Part model, mm, in its own coordinate system. A direction names the side the tool comes from. Give positions to 0.01 mm unless a question says otherwise; leave off trailing zeros. Write each loop counter-clockwise with the first axis right and the second up, starting at its lowest first coordinate (ties: lowest second). Pieces come first, ordered by that corner, then holes. Notation, with made-up numbers: M 13,40.25 L 57,40.25 A18 cw 57,74.25 Z; hole C 2,47 d1. An arc over 180 degrees is marked long. Answer as CSV lines item,"result". Start each with the question number.
Item 1: Band-saw the part on A-A, the plane x = -13.5. List the corners of the cut face in (y, z), then the cut area to 3 significant figures.
Item 2: Pin check, flat tips, straight feed: pin 1 (1 mm diameter, centred on x = -52.5, z = -3.5, fed in from +Y); pin 2 (0.5 mm diameter, centred on x = -25.5, z = -3.5, fed in from -Y); pin 3 (11.5 mm diameter, centred on x = -26, y = -10.5, fed in from +Z); pin 4 (0.6 mm diameter, centred on x = -25, y = 8.5, fed in from +Z). Stop position of each tip, or through.
Item 3: Two-plate mould, pull along Z, no slides. Class faces 1 (the flat face through (-52.292, -33.704, -1.014)), 2 (the flat face through (-27, 17, -2)), 3 (the flat face through (-68, 13, -4)): +Z half, -Z half, draft (parallel to the pull), parting line (faces both ways), or undercut.
Item 4: Band-saw the part on C-C, the plane y = 13. List the corners of the cut face in (x, z).
Item 5: Wall check: L1, parallel to X at y = -2, z = -2.35; L2, parallel to Y at x = -34, z = -2; L3, parallel to Y at x = -32.5, z = -1.25. Give the ranges that are in metal, low to high. Write a range as from..to.
Item 6: Band-saw the part on D-D, the plane y = -18.5. List the corners of the cut face in (x, z), then the cut area to 3 significant figures.
Item 7: 3-axis set-ups, long thin cutter, end or side, ignore diameter. For faces 4 (the flat face through (-26, 0, -1)), 5 (the flat face through (-41, -12, 0)), 6 (the cylindrical face through (-18.29, -2.37, -1.97)): which of +Z, -Z, +X, -X, +Y, -Y reach the whole face in a straight line?
Item 8: Band-saw the part on B-B, the plane y = -34. List the corners of the cut face in (x, z), then the cut area to 3 significant figures.
from build123d import *

# Parameters (mm, degrees)
EXTRUDE_1_DEPTH              = 3
EXTRUDE_2_DEPTH              = 2
FILLET_1_R                   = 2
FILLET_2_R                   = 3
CHAMFER_1_SIZE               = 1
EXTRUDE_3_DEPTH              = 54
PATTERN_LINEAR_1_COUNT       = 4
PATTERN_LINEAR_1_PITCH       = 15
HOLE_WIZARD_M2_2_D           = 1.6
HOLE_WIZARD_M2_2_DEPTH       = 4
HOLE_WIZARD_M2_2_CSINK_D     = 3
HOLE_WIZARD_M2_2_CSINK_ANGLE = 90
PATTERN_LINEAR_2_COUNT       = 3
PATTERN_LINEAR_2_PITCH       = 23
CUT_EXTRUDE_1_DEPTH          = 13
FILLET_3_R                   = 1
CUT_EXTRUDE_2_DEPTH          = 13
FILLET_4_R                   = 1
SKETCH_11_W                  = 2.000000000000007
SKETCH_11_H                  = 5
CUT_EXTRUDE_3_DEPTH          = 1


# Some blends are built 0.0001 mm under size
with BuildPart() as part:
    # 草图1 → 凸台-拉伸1 (new body)
    with BuildSketch(Plane.XY):
        with BuildLine():
            Line((-53, -8.000000000000004), (-53, -14.620000000000001))
            Line((-53, -14.620000000000001), (-54, -14.620000000000001))
            Line((-54, -14.620000000000001), (-54, -39.62))
            Line((-54, -39.62), (-45.9979252690319, -35.00000000000001))
            Line((-45.9979252690319, -35.00000000000001), (-39.02479757997029, -7.032312417601319))
            ThreePointArc((-39.02479757997029, -7.032312417601319), (-37.606260576168935, -4.847956985573115), (-35.14361467486631, -4.000000000000005))
            Line((-35.14361467486631, -4.000000000000005), (4.9e-16, -4))
            Line((4.9e-16, -4), (0, 0))
            Line((0, 0), (-53, 0))
            Line((-53, 0), (-53, -8.000000000000004))
        make_face()
    extrude(amount=-EXTRUDE_1_DEPTH)

    # 草图2 → 凸台-拉伸2 (add)
    with BuildSketch(Plane(origin=(0, 0, -3), x_dir=(-1, 0, 0), z_dir=(0, 0, -1))):
        with BuildLine():
            Line((-4.9e-16, -4), (53, -4))
            Line((53, -4), (53, 6.000000000000002))
            Line((53, 6.000000000000002), (68, 6.000000000000002))
            Line((68, 6.000000000000002), (68, 21))
            Line((68, 21), (65.97847727, 21.000000000000004))
            ThreePointArc((65.97847727, 21.000000000000004), (64.40463560690391, 29.57899182713432), (60.50330893032099, 37.379999999999995))
            Line((60.50330893032099, 37.379999999999995), (60.503308930321, 26.379999999999995))
            Line((60.503308930321, 26.379999999999995), (61.003308930321, 26.38))
            Line((61.003308930321, 26.38), (61.003308930321005, 21))
            Line((61.003308930321005, 21), (53, 21))
            Line((53, 21), (0, 21))
            Line((0, 21), (-4.9e-16, -4))
        make_face()
    extrude(amount=EXTRUDE_2_DEPTH)

    # 圆角1
    fillet_1_edges = [part.edges().sort_by_distance(p)[0] for p in [
        (-44.07180733743316, -4, -3),
    ]]
    fillet(fillet_1_edges, radius=FILLET_1_R - 0.0001)  # a hair under: the kernel refuses the full size

    # 圆角2
    # the kernel refuses this fillet: 3 mm, written as the material it adds along each edge
    with BuildSketch(Plane(origin=(-65.97847727, 21.000000000000004, -3), x_dir=(-1, -3.51e-15, 0), z_dir=(0, 0, -1))) as fillet_2_piece_1:
        with BuildLine():
            CenterArc((2.7704921372998013, 2.9050034125503172), FILLET_2_R, 187.01700367904854, 68.52581158586304)
            Line((-0.2070376849391327, 2.5385117241346675), (-0.2665882813839122, 2.531181890366354))
            ThreePointArc((-0.2665882813839122, 2.531181890366354), (-0.13723895323484658, 1.2665056940841235), (-0.05995131454466218, -0.00241658526998755))
            Line((-0.05995131454466218, -0.00241658526998755), (2.1e-16, -0.05999999999999872))
            ThreePointArc((2.1e-16, -0.05999999999999872), (1.0107613649999936, -0.05999999999999517), (2.006543341853998, -0.05810006825100805))
            Line((2.006543341853998, -0.05810006825100805), (2.021522730000001, 0))
        make_face()
    extrude(amount=2)

    # 倒角1
    chamfer_1_edges = [part.edges().sort_by_distance(p)[0] for p in [
        (-53, -14.620000000000001, -1.5),
    ]]
    chamfer(chamfer_1_edges, length=CHAMFER_1_SIZE - 0.0001)  # a hair under: the kernel refuses the full size

    # 草图3 → 凸台-拉伸3 (add)
    with BuildSketch(Plane(origin=(0, 0, 0), x_dir=(0, 0, -1), z_dir=(1, 1.2e-16, 0))):
        Polygon((1.3e-15, 17), (1.73e-15, 14.000000000000002), (-1.3989229744649714, 17), (-1.3989229744649718, 21), (3, 21), (3.0000000000000018, 17), align=None)
    extrude(amount=-EXTRUDE_3_DEPTH)

    # 草图6 → M2 螺纹孔1 (revolve, cut)
    with BuildSketch(Plane(origin=(-4, -1.9999999999999967, 0), x_dir=(0, -1, 0), z_dir=(1, 0, 0))):
        Polygon((0, 0), (-1.1e-15, 4.480688495222049), (0.7999999999999986, 4), (0.7999999999999899, -1.46e-15), align=None)
    hole_wizard_m2_1 = revolve(axis=Axis((-4, -1.9999999999999967, 6.349999999999991), (0, 0, -1)), mode=Mode.SUBTRACT)

    # 阵列(线性)1: M2 螺纹孔1 ×4
    with Locations(*[(-i * PATTERN_LINEAR_1_PITCH, 0, 0) for i in range(1, PATTERN_LINEAR_1_COUNT)]):
        add(hole_wizard_m2_1, mode=Mode.SUBTRACT)

    # M2 螺纹孔2
    with Locations(Plane(origin=(0, 21, 0), x_dir=(1, 0, 0), z_dir=(0, 1, 0))):
        with Locations((-5, 1.5)):
            hole_wizard_m2_2 = CounterSinkHole(HOLE_WIZARD_M2_2_D / 2, HOLE_WIZARD_M2_2_CSINK_D / 2, depth=HOLE_WIZARD_M2_2_DEPTH, counter_sink_angle=HOLE_WIZARD_M2_2_CSINK_ANGLE)

    # 阵列(线性)2: M2 螺纹孔2 ×3
    with Locations(*[(-i * PATTERN_LINEAR_2_PITCH, 0, 0) for i in range(1, PATTERN_LINEAR_2_COUNT)]):
        add(hole_wizard_m2_2, mode=Mode.SUBTRACT)

    # 草图9 → 切除-拉伸1 (cut)
    with BuildSketch(Plane(origin=(3.89e-15, 37.37999999999999, 7.21e-15), x_dir=(1, -1e-16, 0), z_dir=(1e-16, 1, 1.9e-16))):
        Polygon((-60.503308930321, 4.000000000000004), (-62.23535973788988, 5.000000000000007), (-60.503308930321, 5.000000000000007), align=None)
    extrude(amount=-CUT_EXTRUDE_1_DEPTH, mode=Mode.SUBTRACT)

    # 圆角3
    # the kernel refuses this fillet: 1 mm, written as the material it adds along each edge
    with BuildSketch(Plane(origin=(-58.8382454208599, 24.379999999999995, -3.0386751345948144), x_dir=(1.6e-16, 1, 9e-17), z_dir=(-0.8660254037844387, 0, -0.5))) as fillet_3_piece_1_section:
        with BuildLine():
            CenterArc((FILLET_3_R, FILLET_3_R), FILLET_3_R, 179.99999999999997, 90)
            Line((0, FILLET_3_R), (0, 0))
            Line((0, 0), (FILLET_3_R, 0))
        make_face()
    fillet_3_piece_1 = extrude(amount=6.422649730810377, mode=Mode.PRIVATE)
    fillet_3_piece_1 = split(fillet_3_piece_1, bisect_by=Plane(origin=(-61.495158067637725, 24.669870904160934, -5), z_dir=(0, 0, 1)), keep=Keep.TOP, mode=Mode.PRIVATE)
    fillet_3_piece_1 = split(fillet_3_piece_1, bisect_by=Plane(origin=(-61.003308930321, 24.669870904160934, -4.716030766640193), z_dir=(-1, 1.32e-15, 0)), keep=Keep.TOP, mode=Mode.PRIVATE)
    add(fillet_3_piece_1)

    # 草图10 → 切除-拉伸2 (cut)
    with BuildSketch(Plane(origin=(0, -39.62, 0), x_dir=(1, 0, 0), z_dir=(0, 1, 0))):
        Polygon((-54, 2), (-50.53589838486226, 0), (-54, 1.73e-15), align=None)
    extrude(amount=CUT_EXTRUDE_2_DEPTH, mode=Mode.SUBTRACT)

    # 圆角4
    fillet_4_edges = [part.edges().sort_by_distance(p)[0] for p in [
        (-52.26794919243113, -26.619999999999997, -1),
    ]]
    fillet(fillet_4_edges, radius=FILLET_4_R)

    # 草图11 → 切除-拉伸3 (cut)
    with BuildSketch(Plane.XY.offset(-3)):
        with Locations((-25, 8.5)):
            Rectangle(SKETCH_11_W, SKETCH_11_H)
    extrude(amount=-CUT_EXTRUDE_3_DEPTH, mode=Mode.SUBTRACT)


solid = part.part
Output:
1,outline,"M -4,-5 L 21,-5 L 21,1.4 L 17,1.4 L 14,0 L 17,0 L 17,-3 L 0,-3 L 0,0 L -4,0 Z"
1,area,"81.7 mm²"
2,pin 1,"y = 21"
2,pin 2,"y = -4"
2,pin 3,"through"
2,pin 4,"z = -4"
3,face 1,"+Z half"
3,face 2,"undercut"
3,face 3,"draft"
4,outline,"M -68,-5 L 0,-5 L 0,-3 L -68,-3 Z"
5,L1,"-53..-49.8, -48.2..-34.8, -33.2..-19.8, -18.2..-4.8, -3.2..0"
5,L2,"-4..-2.8, -1.2..0, 17..21"
5,L3,"-4..0, 17..21"
6,outline,"M -54,-3 L -41.88,-3 L -41.88,0 L -54,0 Z"
6,area,"36.3 mm²"
7,face 4,"+Z, +X, -X"
7,face 5,"+Z, +X, -X, -Y"
7,face 6,"+Z"
8,outline,"M -54,-3 L -45.75,-3 L -45.75,0 L -50.54,0 L -54,-2 Z"
8,area,"21.3 mm²"
